```python
from build123d import *

# Parameters (mm, degrees)
SKETCH1_W                = 22.4
SKETCH1_H                = 12.5
BOSS_EXTRUDE1_DEPTH      = 11.4
SKETCH2_R                = 5.63
SKETCH2_R_2              = 2.5
BOSS_EXTRUDE2_DEPTH      = 3.2
BOSS_EXTRUDE3_DEPTH      = 6.25
BOSS_EXTRUDE3_DEPTH_BACK = 6.25
SKETCH3_W                = 31.8
SKETCH3_H                = 2
SKETCH4_R                = 1
CUT_EXTRUDE1_DEPTH       = 25.889405377
CUT_EXTRUDE2_DEPTH       = 25.889405377
SKETCH6_R                = 2.6
BOSS_EXTRUDE4_DEPTH      = 2.6
FILLET1_R                = 1


with BuildPart() as part:
    # Sketch1 → Boss-Extrude1 (new, symmetric)
    with BuildSketch(Plane(origin=(0, 0, 0), x_dir=(1, 0, 0), z_dir=(0, 1, 0))):
        Rectangle(SKETCH1_W, SKETCH1_H)
    extrude(amount=BOSS_EXTRUDE1_DEPTH, both=True)

    # Sketch2 → Boss-Extrude2 (add)
    with BuildSketch(Plane(origin=(0, 11.4, 0), x_dir=(1, 0, 0), z_dir=(0, 1, 0))):
        with Locations((-4.45, 0)):
            Circle(SKETCH2_R)
        with Locations((1.18, 0)):
            Circle(SKETCH2_R_2)
    extrude(amount=BOSS_EXTRUDE2_DEPTH)

    # Sketch3 → Boss-Extrude3 (add, two sides: drawn at the far end of the back side and taken through both)
    with BuildSketch(Plane.XY.offset(-BOSS_EXTRUDE3_DEPTH_BACK)):
        with Locations((0, 5.7)):
            Rectangle(SKETCH3_W, SKETCH3_H)
    extrude(amount=BOSS_EXTRUDE3_DEPTH + BOSS_EXTRUDE3_DEPTH_BACK)

    # Sketch4 → Cut-Extrude1 (cut, through all)
    with BuildSketch(Plane(origin=(0, 6.7, 0), x_dir=(1, 0, 0), z_dir=(0, 1, 0))):
        with Locations(Location((-13.85, 0, 0), (0, 0, 270))):
            Circle(SKETCH4_R)
        with Locations(Location((13.85, 0, 0), (0, 0, 270))):
            Circle(SKETCH4_R)
    extrude(amount=-CUT_EXTRUDE1_DEPTH, mode=Mode.SUBTRACT)

    # Sketch5 → Cut-Extrude2 (cut, through all)
    with BuildSketch(Plane(origin=(0, 6.7, 0), x_dir=(1, 0, 0), z_dir=(0, 1, 0))):
        with BuildLine():
            Line((-17.95, 0.4), (-13.85, 0.4))
            ThreePointArc((-13.85, 0.4), (-13.45, 0), (-13.85, -0.4))
            Line((-13.85, -0.4), (-17.95, -0.4))
            ThreePointArc((-17.95, -0.4), (-18.35, 0), (-17.95, 0.4))
        make_face()
        with BuildLine():
            Line((17.95, -0.4), (13.85, -0.4))
            ThreePointArc((13.85, -0.4), (13.45, 0), (13.85, 0.4))
            Line((13.85, 0.4), (17.95, 0.4))
            ThreePointArc((17.95, 0.4), (18.35, 0), (17.95, -0.4))
        make_face()
    extrude(amount=-CUT_EXTRUDE2_DEPTH, mode=Mode.SUBTRACT)

    # Sketch6 → Boss-Extrude4 (add)
    with BuildSketch(Plane(origin=(0, 14.6, 0), x_dir=(1, 0, 0), z_dir=(0, 1, 0))):
        with Locations(Location((-4.45, 0, 0), (0, 0, 270))):
            Circle(SKETCH6_R)
    extrude(amount=BOSS_EXTRUDE4_DEPTH)

    # Fillet1
    fillet1_edges = [part.edges().sort_by_distance(p)[0] for p in [
        (11.2, -3.35, 6.25),
        (-11.2, -3.35, 6.25),
        (-11.2, -3.35, -6.25),
        (11.2, -3.35, -6.25),
        (15.9, 5.7, 6.25),
        (-15.9, 5.7, 6.25),
        (-15.9, 5.7, -6.25),
        (15.9, 5.7, -6.25),
        (11.2, 9.05, 6.25),
        (-11.2, 9.05, 6.25),
        (-11.2, 9.05, -6.25),
        (11.2, 9.05, -6.25),
    ]]
    fillet(fillet1_edges, radius=FILLET1_R)

    # Sweep1: sweep along a path in Sketch8
    with BuildLine(Plane.XY) as sweep1_path:
        Line((-11.2, -7.4), (-12.7, -7.4))
        ThreePointArc((-12.7, -7.4), (-14.936067977, -8.781966011), (-14.7, -11.4))
    # Sketch7 → Sweep1 (sweep)
    with BuildSketch(Plane.ZY.offset(11.2)):
        with BuildLine():
            ThreePointArc((0.25, -6.966987298), (0, -6.9), (-0.25, -6.966987298))
            ThreePointArc((-0.25, -6.966987298), (-1, -7.4), (-0.25, -7.833012702))
            ThreePointArc((-0.25, -7.833012702), (0, -7.9), (0.25, -7.833012702))
            ThreePointArc((0.25, -7.833012702), (1, -7.4), (0.25, -6.966987298))
        make_face()
    sweep(path=sweep1_path.line)


solid = part.part
```
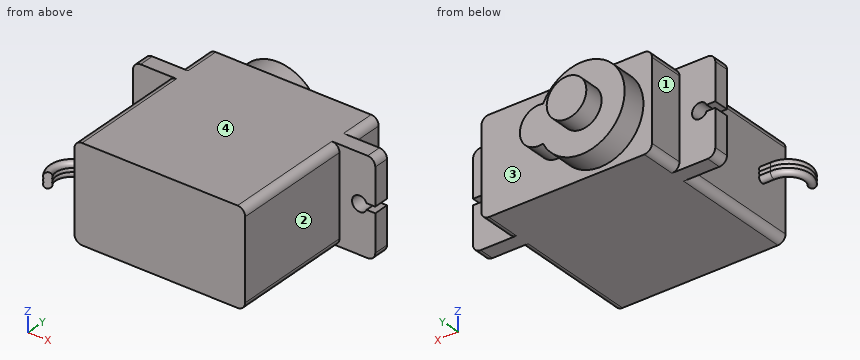
Verification items for the finished model (mm, model axes). Face numbers are marked on the shaded views. A direction names the side the tool comes from. Round coordinates to 2 decimals unless told otherwise and drop trailing zeros. Write each loop counter-clockwise with the first axis right and the second up, starting at its lowest first coordinate (ties: lowest second). Pieces come first, ordered by that corner, then holes. Notation, with made-up numbers: (-14.75, 0) - (-3.75, 0) arc R30 cw to (-3.75, 30) - close; hole circle Ø8 at (-4, 75). An arc over 180 degrees is marked (long way). Answer as a JSON object with one key per item and string values. Group by question number.
Q1. Section check C-C, the plane x = -4.45. Enter the section's corners in (y, z), plus the area to 3 significant figures.
Q2. Section check D-D, the plane z = 2. Enter the section's corners in (x, y), plus the area to 3 significant figures.
Q3. Section check A-A, the plane x = 13.85. Enter the section's corners in (y, z).
Q4. Tool access check on the marked faces 1, 2, 3 and 4. Record the directions out of +Z, -Z, +X, -X, +Y, -Y that give a thin tool (end or side, any length) a straight path to the whole face; none if there is none.
Q5. Section check B-B, the plane y = 10. Enter the section's corners in (x, z).
Q6. Go/stop test with flat-tipped pins: pin 1 Ø4.5 at (x, z) = (13, -3) entering from +Y; pin 2 Ø2.5 at (x, z) = (13.85, 0) entering from -Y; pin 3 Ø5 at (y, z) = (0.5, -2) entering from +X; pin 4 Ø0.9 at (x, y) = (-15, 5.5) entering from +Z. Record where each tip stops, or that it passes through.
Q7. Thickness scan on line 1 (Z direction, x = 13.85, y = 6.1); line 2 (X direction, y = -5.25, z = -0.5); line 3 (X direction, y = 6.1, z = 0). Record the ranges inside material, lowest first.
Found:
{
 "1": {"outline": "(-11.4, -6.25) - (11.4, -6.25) - (11.4, -5.63) - (14.6, -5.63) - (14.6, -2.6) - (17.2, -2.6) - (17.2, 2.6) - (14.6, 2.6) - (14.6, 5.63) - (11.4, 5.63) - (11.4, 6.25) - (-11.4, 6.25) - close", "area": "335 mm^2"},
 "2": {"outline": "(-15.9, 4.7) - (-11.2, 4.7) - (-11.2, -11.4) - (11.2, -11.4) - (11.2, 4.7) - (15.9, 4.7) - (15.9, 6.7) - (11.2, 6.7) - (11.2, 11.4) - (2.68, 11.4) - (2.68, 14.6) - (-2.79, 14.6) - (-2.79, 17.2) - (-6.11, 17.2) - (-6.11, 14.6) - (-9.71, 14.6) - (-9.71, 11.4) - (-11.2, 11.4) - (-11.2, 6.7) - (-15.9, 6.7) - close", "area": "578 mm^2"},
 "3": {"outline": "(4.7, -6.25) - (6.7, -6.25) - (6.7, -1) - (4.7, -1) - close; (4.7, 1) - (6.7, 1) - (6.7, 6.25) - (4.7, 6.25) - close"},
 "4": {"face 1": "+Z, -Z, -X, +Y", "face 2": "+Z, -Z, +X, -Y", "face 3": "+Y", "face 4": "+Z, +X, -X, +Y, -Y"},
 "5": {"outline": "(-11.2, -5.25) arc R1 ccw to (-10.2, -6.25) - (10.2, -6.25) arc R1 ccw to (11.2, -5.25) - (11.2, 5.25) arc R1 ccw to (10.2, 6.25) - (-10.2, 6.25) arc R1 ccw to (-11.2, 5.25) - close"},
 "6": {"pin 1": "stops at y = 11.4", "pin 2": "stops at y = 4.7", "pin 3": "stops at x = 11.2", "pin 4": "stops at z = 6.25"},
 "7": {"line 1": "z = -6.25 to -1, 1 to 6.25", "line 2": "x = -11.2 to 11.2", "line 3": "x = -12.85 to 12.85"}
}
